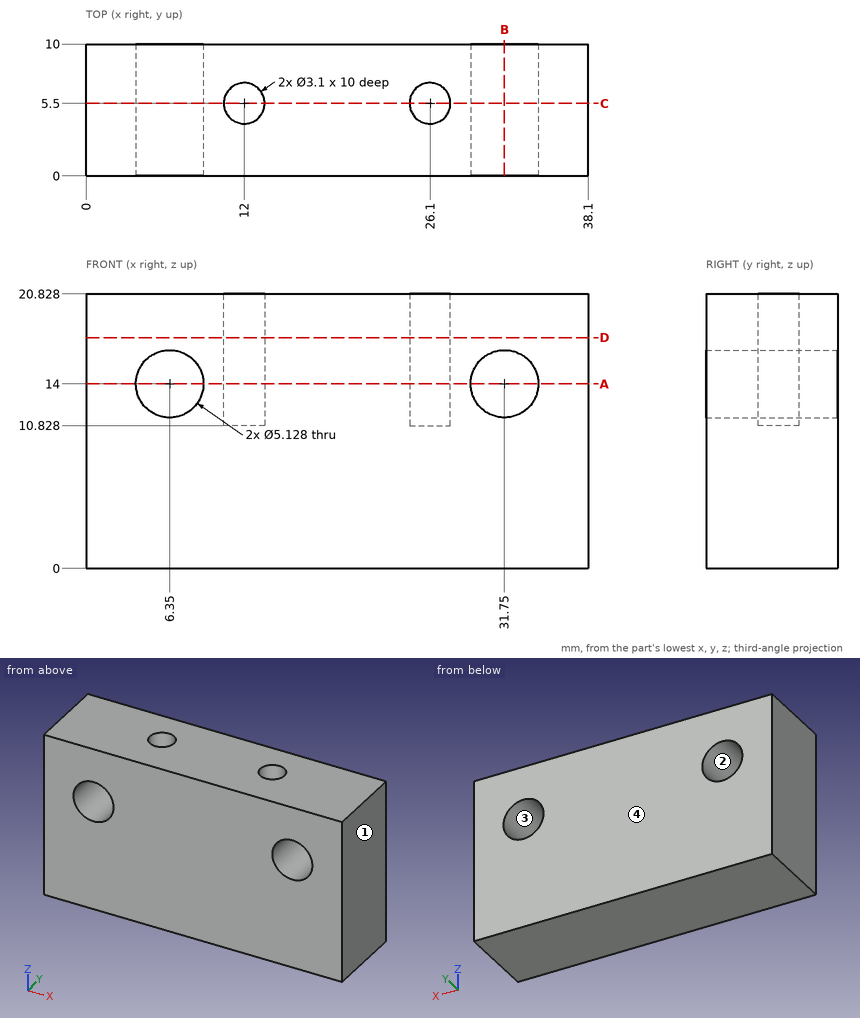
The figure shows three views and two pictorial views of one solid part (mm, origin at its lowest corner). Answer the questions. Give positions to 0.01 mm unless a question says otherwise; leave off trailing zeros. Order: outer loops, then holes, each group sorted by start corner. A loop starts at its lowest first (then second) coordinate and runs counter-clockwise, first axis right, second up. Notation, with made-up numbers: (50.25, 80.25) -> (107.25, 80.25) arc R9 cw to (107.25, 89.25) -> close; hole circle Ø6 at (81.5, 54). An arc over 180 degrees is marked (long way). Answer as CSV lines item,"result". Start each with the question number.
(1) Each of these flat-tipped pins is pushed along its axis until it touches: pin 1 Ø1.9 at (x, y) = (12, 5.5) entering from +Z; pin 2 Ø4 at (x, z) = (31.75, 14) entering from +Y. Where does it stop, or does it pass through?
(2) For a pull along X with two mould halves and no side action, classify the marked faces 1, 2, 3 and 4 as released by +X, released by -X, zero draft, split by the parting line, or undercut.
(3) Section D-D, the plane z = 17.5 is taken. Write down the section's boundary in (x, y).
(4) Section A-A, the plane z = 14 is taken. Write down the section's boundary in (x, y), plus the area to 3 significant figures.
(5) Consider line 1 along Y through (x, z) = (26.1, 18.25); line 2 along X through (y, z) = (6.75, 14); line 3 along X through (y, z) = (9.75, 13.5). Determine where each line is inside the solid, lowest interval first.
(6) Section B-B, the plane x = 31.75 is taken. Write down the section's boundary in (y, z).
(7) Section C-C, the plane y = 5.5 is taken. Write down the section's boundary in (x, z), plus the area to 3 significant figures.
Entries:
1,pin 1,"z = 10.83"
1,pin 2,"through"
2,face 1,"released by +X"
2,face 2,"undercut"
2,face 3,"undercut"
2,face 4,"zero draft"
3,outline,"(0, 0) -> (38.1, 0) -> (38.1, 10) -> (0, 10) -> close; hole circle Ø3.1 at (12, 5.5); hole circle Ø3.1 at (26.1, 5.5)"
4,outline,"(0, 0) -> (3.79, 0) -> (3.79, 10) -> (0, 10) -> close; (8.91, 0) -> (29.19, 0) -> (29.19, 10) -> (8.91, 10) -> close; (34.31, 0) -> (38.1, 0) -> (38.1, 10) -> (34.31, 10) -> close; hole circle Ø3.1 at (12, 5.5); hole circle Ø3.1 at (26.1, 5.5)"
4,area,"263 mm²"
5,line 1,"0 to 3.95, 7.05 to 10"
5,line 2,"0 to 3.79, 8.91 to 11.08, 12.92 to 25.18, 27.02 to 29.19, 34.31 to 38.1"
5,line 3,"0 to 3.84, 8.86 to 29.24, 34.26 to 38.1"
6,outline,"(0, 0) -> (10, 0) -> (10, 11.44) -> (0, 11.44) -> close; (0, 16.56) -> (10, 16.56) -> (10, 20.83) -> (0, 20.83) -> close"
7,outline,"(0, 0) -> (38.1, 0) -> (38.1, 20.83) -> (27.65, 20.83) -> (27.65, 10.83) -> (24.55, 10.83) -> (24.55, 20.83) -> (13.55, 20.83) -> (13.55, 10.83) -> (10.45, 10.83) -> (10.45, 20.83) -> (0, 20.83) -> close; hole circle Ø5.13 at (6.35, 14); hole circle Ø5.13 at (31.75, 14)"
7,area,"690 mm²"
